Study the drawing (mm; zero at the part's minimum x, y, z) and answer. A direction names the side the tool comes from. Round coordinates to 2 decimals unless told otherwise and drop trailing zeros. Loops run counter-clockwise (first coordinate to the right, second up) from the corner with the lowest first, then second, coordinate; pieces in that order, holes last. Notation, with made-up numbers: (-35, -17) -> (9, -17) arc R11 cw to (9, -4) -> close; hole circle Ø1 at (52.25, 61). An arc over 180 degrees is marked (long way). Write each question's results on one line, items separated by ' | '. Start each with the question number.
(1) Determine the mould class of the marked faces 3, 4 and 5 for opening direction Z: released by +Z, released by -Z, zero draft, split by the parting line, or undercut.
(2) Flat-ended cylindrical pins translate along their axes: pin 1 (1 mm diameter, centred on y = 4, z = 4.5, fed in from -X); pin 2 (0.9 mm diameter, centred on x = 2.5, z = 3.125, fed in from -Y). Find the tip coordinate at first contact, or state that the pin passes through.
(3) For the marked faces 1 and 2, determine the directions among +Z, -Z, +X, -X, +Y, -Y from which every point of the face is accessible in a straight line to the end or side of a thin tool.
(4) The part is cut by section D-D (x = 12.5). Determine the outline of the cut face in (y, z) (3 decimals), plus the area to 4 significant figures.
(5) The part is cut by section B-B (z = 5.25). Determine the outline of the cut face in (x, y) (3 decimals), plus the area to 3 significant figures.
(6) Straight lines are drawn through the part: probe 1 along X at (y, z) = (3.15, 4); probe 2 along Y at (x, z) = (6.25, 0.5) (3 decimals); probe 3 along X at (y, z) = (3.45, 3). For each, find the intervals that lie inside material, in ascending order.
(7) The part is cut by section C-C (y = 2.7). Determine the outline of the cut face in (x, z) (3 decimals), plus the area to 3 significant figures.
(8) The part is cut by section A-A (x = 9.5). Determine the outline of the cut face in (y, z) (3 decimals), plus the area to 3 significant figures.
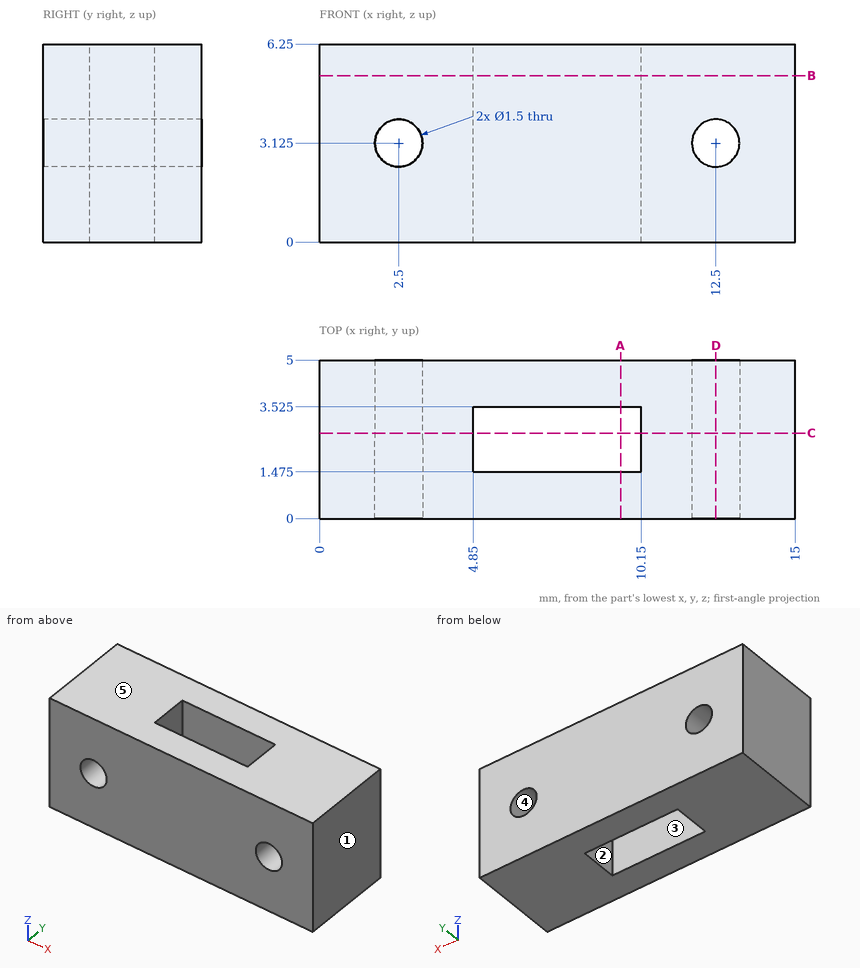
Checked values:
1) face 3: zero draft | face 4: undercut | face 5: released by +Z
2) pin 1: stops at x = 0 | pin 2: passes through
3) face 1: +Z, -Z, +X, +Y, -Y | face 2: +Z, -Z
4) outline: (0, 0) -> (5, 0) -> (5, 2.375) -> (0, 2.375) -> close; (0, 3.875) -> (5, 3.875) -> (5, 6.25) -> (0, 6.25) -> close | area: 23.75 mm2
5) outline: (0, 0) -> (15, 0) -> (15, 5) -> (0, 5) -> close; hole (4.85, 1.475) -> (10.15, 1.475) -> (10.15, 3.525) -> (4.85, 3.525) -> close | area: 64.1 mm2
6) probe 1: x = 0 to 4.85, 10.15 to 15 | probe 2: y = 0 to 1.475, 3.525 to 5 | probe 3: x = 0 to 1.76, 3.24 to 4.85, 10.15 to 11.76, 13.24 to 15
7) outline: (0, 0) -> (4.85, 0) -> (4.85, 6.25) -> (0, 6.25) -> close; (10.15, 0) -> (15, 0) -> (15, 6.25) -> (10.15, 6.25) -> close; hole circle Ø1.5 at (2.5, 3.125); hole circle Ø1.5 at (12.5, 3.125) | area: 57.1 mm2
8) outline: (0, 0) -> (1.475, 0) -> (1.475, 6.25) -> (0, 6.25) -> close; (3.525, 0) -> (5, 0) -> (5, 6.25) -> (3.525, 6.25) -> close | area: 18.4 mm2
